Read the model definition and answer for the solid it produces. Units are mm, in the model's axes. A direction names the side the tool comes from. Give positions to 0.01 mm unless a question says otherwise; leave off trailing zeros. Order: outer loops, then holes, each group sorted by start corner. A loop starts at its lowest first (then second) coordinate and runs counter-clockwise, first axis right, second up. Notation, with made-up numbers: (79.5, 44.5) - (88.5, 44.5) arc R27 cw to (88.5, 66.5) - close; hole circle Ø2 at (86, 50). An arc over 180 degrees is marked (long way). Return JSON: item names as keys, results as strings.
```python
from build123d import *

# Parameters (mm, degrees)
EXTRUDE_1_DEPTH     = 15
CUT_EXTRUDE_1_DEPTH = 5
SKETCH_3_R          = 1.6
SKETCH_3_W          = 5
SKETCH_3_H          = 5
CUT_EXTRUDE_2_DEPTH = 22
FILLET_1_R          = 2
SKETCH_4_W          = 9.58124175
SKETCH_4_H          = 10
EXTRUDE_2_DEPTH     = 17
SKETCH_5_R          = 1.6
CUT_EXTRUDE_3_DEPTH = 18
FILLET_2_R          = 3


with BuildPart() as part:
    # 草图1 → 凸台-拉伸1 (new body)
    with BuildSketch(Plane.XY):
        with BuildLine():
            Line((24.185160084, -7.016301696), (24.496510845, 5.979969335))
            ThreePointArc((24.496510845, 5.979969335), (23.944762934, 7.407806858), (22.544984649, 8.027295764))
            Line((22.544984649, 8.027295764), (-13.444688974, 8.889497871))
            Line((-13.444688974, 8.889497871), (-13.265063535, 16.387346543))
            Line((-13.265063535, 16.387346543), (-18.263629316, 16.507096835))
            ThreePointArc((-18.263629316, 16.507096835), (-21.833223125, 15.127727058), (-23.38194539, 11.628281347))
            Line((-23.38194539, 11.628281347), (-23.908846678, -10.36540809))
            ThreePointArc((-23.908846678, -10.36540809), (-22.5294769, -13.935001898), (-19.030031189, -15.483724163))
            Line((-19.030031189, -15.483724163), (-14.031465408, -15.603474456))
            Line((-14.031465408, -15.603474456), (-13.851839969, -8.105625784))
            Line((-13.851839969, -8.105625784), (22.137833654, -8.967827891))
            ThreePointArc((22.137833654, -8.967827891), (23.565671178, -8.41607998), (24.185160084, -7.016301696))
        make_face()
        with BuildLine():
            ThreePointArc((-16.75044735, -12.037331753), (-18.893602347, -9.788969482), (-21.141964619, -11.93212448))
            ThreePointArc((-21.141964619, -11.93212448), (-18.998809621, -14.180486751), (-16.75044735, -12.037331753))
        make_face(mode=Mode.SUBTRACT)
        with BuildLine():
            ThreePointArc((-16.04728092, -4.552025517), (-18.701434473, -1.76757982), (-21.48588017, -4.421733373))
            ThreePointArc((-21.48588017, -4.421733373), (-18.831726617, -7.20617907), (-16.04728092, -4.552025517))
        make_face(mode=Mode.SUBTRACT)
        with BuildLine():
            ThreePointArc((-15.807780335, 5.445106045), (-18.461933888, 8.229551742), (-21.246379585, 5.575398189))
            ThreePointArc((-21.246379585, 5.575398189), (-18.592226032, 2.790952492), (-15.807780335, 5.445106045))
        make_face(mode=Mode.SUBTRACT)
        with BuildLine():
            ThreePointArc((-16.151695887, 12.955497152), (-18.294850884, 15.203859423), (-20.543213156, 13.060704426))
            ThreePointArc((-20.543213156, 13.060704426), (-18.400058158, 10.812342154), (-16.151695887, 12.955497152))
        make_face(mode=Mode.SUBTRACT)
    extrude(amount=-EXTRUDE_1_DEPTH)

    # 草图2 → 切除-拉伸1 (cut)
    with BuildSketch(Plane(origin=(0, 0, -15), x_dir=(-1, 0, 0), z_dir=(0, 0, -1))):
        Polygon((13.444688974, 8.889497871), (13.851839969, -8.105625784), (-33.415838559, -15.121344773), (-27.379501609, 15.743180277), align=None)
    extrude(amount=-CUT_EXTRUDE_1_DEPTH, mode=Mode.SUBTRACT)

    # 草图3 → 切除-拉伸2 (cut)
    with BuildSketch(Plane(origin=(0.205130979, 8.562490084, 0), x_dir=(0.9997131562086496, -0.02395005852477245, 0), z_dir=(0.02395005852477245, 0.9997131562086496, 0))):
        with Locations(Location((21.846263557, 5, 0), (0, 0, 288.209956864))):
            Circle(SKETCH_3_R)
        with Locations(Location((-8.153736443, 5, 0), (0, 0, 180))):
            Circle(SKETCH_3_R)
        with Locations((9.846263557, 7.5)):
            Rectangle(SKETCH_3_W, SKETCH_3_H)
    extrude(amount=-CUT_EXTRUDE_2_DEPTH, mode=Mode.SUBTRACT)

    # 圆角1
    fillet_1_edges = [part.edges().sort_by_distance(p)[0] for p in [
        (7.142136311, -8.608577013, -7.5),
        (7.549287306, 8.386546642, -7.5),
    ]]
    fillet(fillet_1_edges, radius=FILLET_1_R)

    # 草图4 → 凸台-拉伸2 (add)
    with BuildSketch(Plane(origin=(-0.202020016, -8.432633571, 0), x_dir=(0.9997131562086498, -0.023950058524770876, 0), z_dir=(-0.023950058524770876, -0.9997131562086498, 0))):
        with Locations((24.555642682, -5)):
            Rectangle(SKETCH_4_W, SKETCH_4_H)
    extrude(amount=-EXTRUDE_2_DEPTH)

    # 草图5 → 切除-拉伸3 (cut)
    with BuildSketch(Plane(origin=(-0.202020016, -8.432633571, 0), x_dir=(0.9997131562086498, -0.023950058524770876, 0), z_dir=(-0.023950058524770876, -0.9997131562086498, 0))):
        with Locations((26.846263557, -5)):
            Circle(SKETCH_5_R)
    extrude(amount=-CUT_EXTRUDE_3_DEPTH, mode=Mode.SUBTRACT)

    # 圆角2
    # the kernel refuses this fillet: 3 mm, written as the material it takes off along each edge
    with BuildSketch(Plane(origin=(29.135825748, -9.135478301, 7.5), x_dir=(-0.9997131562086498, 0.023950058524770713, 0), z_dir=(0, 0, -1)), Plane(origin=(29.542976743, 7.859645355, 7.5), x_dir=(-0.023950058524770713, -0.9997131562086498, 0), z_dir=(0, 0, -1))) as fillet_2_piece_1:
        with BuildLine():
            CenterArc((FILLET_2_R, FILLET_2_R), FILLET_2_R, 180, 90)
            Line((0, FILLET_2_R), (0, 0))
            Line((0, 0), (FILLET_2_R, 0))
        make_face()
    extrude(amount=25, mode=Mode.SUBTRACT)


solid = part.part
```
Q1. A cutting plane is placed at D-D (z = -2). Write down the section's boundary in (x, y), and give its area (3 significant figures).
Values:
{"outline": "(-23.91, -10.37) arc R5 ccw to (-19.03, -15.48) - (-14.03, -15.6) - (-13.85, -8.11) - (26.14, -9.06) arc R3 ccw to (29.21, -6.14) - (29.47, 4.86) arc R3 ccw to (26.54, 7.93) - (-13.44, 8.89) - (-13.27, 16.39) - (-18.26, 16.51) arc R5 ccw to (-23.38, 11.63) - close; hole circle Ø5.44 at (-18.77, -4.49); hole circle Ø5.44 at (-18.53, 5.51); hole circle Ø4.39 at (-18.95, -11.98); hole circle Ø4.39 at (-18.35, 13.01)", "area": "960 mm²"}
Q2. A cutting plane is placed at B-B (z = -12). Write down the section's boundary in (x, y).
Values:
{"outline": "(-23.91, -10.37) arc R5 ccw to (-19.03, -15.48) - (-14.03, -15.6) - (-13.27, 16.39) - (-18.26, 16.51) arc R5 ccw to (-23.38, 11.63) - close; hole circle Ø5.44 at (-18.77, -4.49); hole circle Ø5.44 at (-18.53, 5.51); hole circle Ø4.39 at (-18.95, -11.98); hole circle Ø4.39 at (-18.35, 13.01)"}
Q3. Consider L1, parallel to X at y = 6.5, z = -7.5; L2, parallel to X at y = 5.5, z = -4.5; L3, parallel to Z at x = 10, y = 8. Determine where each line is inside the solid, lowest interval first.
Values:
{"L1": "x = -23.5 to -21.06, -15.99 to 7.5, 12.51 to 29.03", "L2": "x = -23.53 to -21.25, -15.81 to -9.54, -6.5 to 25.47, 28.51 to 29.42", "L3": "z = -5 to 0"}
Q4. For faces 1 (the cylindrical face through (28.363, -0.734, -4.519)), 2 (the flat face through (21, 0, -10)), 3 (the cylindrical face through (-16.329, 7.113, -7.395)), determine the directions among +Z, -Z, +X, -X, +Y, -Y from which every point of the face is accessible in a straight line to the end or side of a thin tool.
Values:
{"face 1": "none", "face 2": "-Z, +X, +Y, -Y", "face 3": "+Z, -Z"}
Q5. A cutting plane is placed at A-A (z = -4.25). Write down the section's boundary in (x, y).
Values:
{"outline": "(-23.91, -10.37) arc R5 ccw to (-19.03, -15.48) - (-14.03, -15.6) - (-13.85, -8.11) - (-9.77, -8.2) - (-9.36, 8.79) - (-13.44, 8.89) - (-13.27, 16.39) - (-18.26, 16.51) arc R5 ccw to (-23.38, 11.63) - close; (-6.94, -8.27) - (25.22, -9.04) - (25.63, 7.95) - (-6.53, 8.72) - close; (28.07, -8.42) arc R3 ccw to (29.21, -6.14) - (29.47, 4.86) arc R3 ccw to (28.44, 7.2) - close; hole circle Ø5.44 at (-18.77, -4.49); hole circle Ø5.44 at (-18.53, 5.51); hole circle Ø4.39 at (-18.95, -11.98); hole circle Ø4.39 at (-18.35, 13.01)"}
Q6. Determine the mould class of faces 4 (the cylindrical face through (-20.356, 13.898, -7.395)), 5 (the flat face through (-19, 1, -15)), 6 (the cylindrical face through (28.95, 6.62, -4.93)) for opening direction X: released by +X, released by -X, zero draft, split by the parting line, or undercut.
Values:
{"face 4": "undercut", "face 5": "zero draft", "face 6": "released by +X"}
Q7. Given pin 1 (5 mm diameter, centred on x = -11.5, z = -2, fed in from +Y); pin 2 (14 mm diameter, centred on x = 19.5, y = -1.5, fed in from -Z); pin 3 (8 mm diameter, centred on x = 5, z = -12.5, fed in from +Y), each flat-ended and moving along its own axis, determine where each tip first touches the part or whether it passes through.
Values:
{"pin 1": "stops at y = 16.4", "pin 2": "stops at z = -10", "pin 3": "stops at y = 8.52"}
Q8. A cutting plane is placed at C-C (y = -3). Give the number of separate pieces and of enclosed holes in the cut face, and give its area (3 significant figures).
Values:
{"separate pieces": "2", "enclosed holes": "2", "area": "471 mm²"}
